from build123d import *

# Parameters (mm, degrees)
SKETCH1_W               = 42
SKETCH1_H               = 7
RISER_DEPTH             = 7
SKETCH2_R               = 1.575
MOUNTING_HOLES_DEPTH    = 44.150898021
SKETCH3_W               = 40.15
SKETCH3_H               = 5.15
RECESS_DEPTH            = 3
SKETCH4_W               = 42
SKETCH4_H               = 7
FLANGE_DEPTH            = 7
SKETCH5_W               = 19.5
SKETCH5_H               = 6.925
FLANGE_CUTOUT_DEPTH     = 5
ANGLE_CUTOUT_DEPTH      = 27.594172294
ANGLE_CUTOUT_DEPTH_BACK = 27.594172294
FLANGE_CHAMFER_1_SIZE   = 1
FLANGE_CHAMFER_2_SIZE   = 1


with BuildPart() as part:
    # Sketch1 → Riser (new body)
    with BuildSketch(Plane(origin=(0, 0, 0), x_dir=(1, 0, 0), z_dir=(0, 1, 0))):
        with Locations((21, 3.5)):
            Rectangle(SKETCH1_W, SKETCH1_H)
    extrude(amount=RISER_DEPTH)

    # Sketch2 → Mounting Holes (cut, through all)
    with BuildSketch(Plane.XZ):
        with Locations(Location((5, -3.5, 0), (0, 0, 90))):
            Circle(SKETCH2_R)
        with Locations(Location((37, -3.5, 0), (0, 0, 270))):
            Circle(SKETCH2_R)
    extrude(amount=-MOUNTING_HOLES_DEPTH, mode=Mode.SUBTRACT)

    # Sketch3 → Recess (cut)
    with BuildSketch(Plane(origin=(0, 7, 0), x_dir=(1, 0, 0), z_dir=(0, 1, 0))):
        with Locations((21, 3.5)):
            Rectangle(SKETCH3_W, SKETCH3_H)
    extrude(amount=-RECESS_DEPTH, mode=Mode.SUBTRACT)

    # Sketch4 → Flange (add)
    with BuildSketch(Plane(origin=(0, 0, 0), x_dir=(1, 0, 0), z_dir=(0, 1, 0))):
        with Locations((21, 10.5)):
            Rectangle(SKETCH4_W, SKETCH4_H)
    extrude(amount=FLANGE_DEPTH)

    # Sketch5 → Flange Cutout (cut)
    with BuildSketch(Plane(origin=(0, 7, 0), x_dir=(1, 0, 0), z_dir=(0, 1, 0))):
        with Locations((10.75, 10.5375)):
            Rectangle(SKETCH5_W, SKETCH5_H)
        with Locations((31.25, 10.5375)):
            Rectangle(SKETCH5_W, SKETCH5_H)
    extrude(amount=-FLANGE_CUTOUT_DEPTH, mode=Mode.SUBTRACT)

    # Sketch7 → Angle Cutout (cut, two sides: drawn at the far end of the back side and taken through both)
    with BuildSketch(Plane.ZY.offset(-20.5).offset(-ANGLE_CUTOUT_DEPTH_BACK)):
        Polygon((-7.075, 7), (-14, 2), (-14, 7), align=None)
    extrude(amount=ANGLE_CUTOUT_DEPTH + ANGLE_CUTOUT_DEPTH_BACK, mode=Mode.SUBTRACT)

    # Flange Chamfer 1
    flange_chamfer_1_edges = [part.edges().sort_by_distance(p)[0] for p in [
        (10.75, 2, -7.075),
    ]]
    chamfer(flange_chamfer_1_edges, length=FLANGE_CHAMFER_1_SIZE)

    # Flange Chamfer 2
    flange_chamfer_2_edges = [part.edges().sort_by_distance(p)[0] for p in [
        (31.25, 2, -7.075),
    ]]
    chamfer(flange_chamfer_2_edges, length=FLANGE_CHAMFER_2_SIZE)


solid = part.part
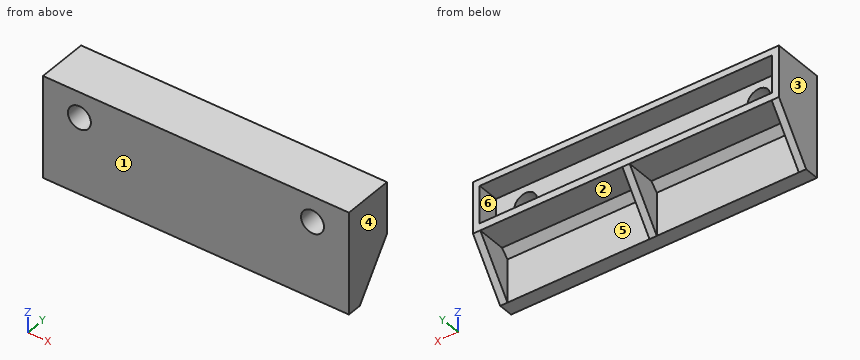
Could you check a few things on this model? Use its own coordinates, in mm. Face numbers are marked on the shaded views. A direction names the side the tool comes from. Round coordinates to 2 decimals unless told otherwise and drop trailing zeros. Loops run counter-clockwise (first coordinate to the right, second up) from the corner with the lowest first, then second, coordinate; pieces in that order, holes last. Notation, with made-up numbers: (-10, -3) -> (31, -3) arc R24 cw to (31, 30) -> close; hole circle Ø2 at (50, 44). An arc over 180 degrees is marked (long way). Use CSV: the item, a comma, the result in double quotes.
(1) Suppose I cut it at C-C on x = 16. Write out the boundary of the cut face in (y, z) (3 decimals), plus the area to 3 significant figures.
Return value:
outline,"(0, -14) -> (2, -14) -> (2, -8.075) -> (3, -7.075) -> (7, -7.075) -> (7, -6.075) -> (4, -6.075) -> (4, -0.925) -> (7, -0.925) -> (7, 0) -> (0, 0) -> close"
area,"48.4 mm²"
(2) If we mould it in two halves opening along X, with no side actions, what happens to the marked faces 1, 2 and 3? For each: +X half, -X half, draft (parallel to the pull), parting line (faces both ways), or undercut.
Return value:
face 1,"draft"
face 2,"undercut"
face 3,"-X half"
(3) Suppose I cut it at A-A on x = 5. Write out the boundary of the cut face in (y, z) (3 decimals).
Return value:
outline,"(0, -14) -> (2, -14) -> (2, -8.075) -> (3, -7.075) -> (7, -7.075) -> (7, -6.075) -> (4, -6.075) -> (4, -5.075) -> (0, -5.075) -> close; (0, -1.925) -> (4, -1.925) -> (4, -0.925) -> (7, -0.925) -> (7, 0) -> (0, 0) -> close"
(4) Suppose I cut it at D-D on y = 5.25. Write out the boundary of the cut face in (x, z) (3 decimals).
Return value:
outline,"(0, -9.499) -> (1, -9.499) -> (1, -7.075) -> (20.5, -7.075) -> (20.5, -9.499) -> (21.5, -9.499) -> (21.5, -7.075) -> (41, -7.075) -> (41, -9.499) -> (42, -9.499) -> (42, 0) -> (0, 0) -> close; hole (0.925, -6.075) -> (41.075, -6.075) -> (41.075, -0.925) -> (0.925, -0.925) -> close"
(5) For the marked faces 4, 5 and 6, which set-ups out of +Z, -Z, +X, -X, +Y, -Y let a thin tool reach every point of the face, with its end or its side?
Return value:
face 4,"+Z, -Z, +X, +Y, -Y"
face 5,"-Z, +Y"
face 6,"+Y"
(6) Suppose I cut it at B-B on z = -3.5. Write out the boundary of the cut face in (x, y) (3 decimals), plus the area to 3 significant figures.
Return value:
outline,"(0, 0) -> (3.425, 0) -> (3.425, 4) -> (0.925, 4) -> (0.925, 7) -> (0, 7) -> close; (6.575, 0) -> (35.425, 0) -> (35.425, 4) -> (6.575, 4) -> close; (38.575, 0) -> (42, 0) -> (42, 7) -> (41.075, 7) -> (41.075, 4) -> (38.575, 4) -> close"
area,"148 mm²"
(7) Will these pins go through, and if not, where does the flat tip stop? pin 1 Ø2.5 at (x, y) = (18.5, 6) entering from -Z (3 decimals); pin 2 Ø1.9 at (x, z) = (5, -3.5) entering from +Y; pin 3 Ø1.5 at (x, z) = (24, -3.5) entering from +Y; pin 4 Ø4.5 at (x, z) = (7, -12.5) entering from +Y.
Return value:
pin 1,"stops at z = -7.075"
pin 2,"passes through"
pin 3,"stops at y = 4"
pin 4,"stops at y = 2"
(8) If I drill on probe 1 along X at (y, z) = (1.65, -3.5) (3 decimals); probe 2 along X at (y, z) = (2.5, -8); probe 3 along Z at (x, y) = (35.5, 6.75) (3 decimals), over which ranges is the centre line in solid material (lowest first)? Write a range as [from, to].
Return value:
probe 1,"x = [0, 3.425], [6.575, 35.425], [38.575, 42]"
probe 2,"x = [0, 1], [20.5, 21.5], [41, 42]"
probe 3,"z = [-7.075, -6.075], [-0.925, 0]"
